Could you check a few things on this model? Use its own coordinates, in mm. A direction names the side the tool comes from. Give positions to 0.01 mm unless a question says otherwise; leave off trailing zeros. Write each loop counter-clockwise with the first axis right and the second up, starting at its lowest first coordinate (ties: lowest second). Pieces come first, ordered by that corner, then holes. Notation, with made-up numbers: M -17,72 L 4,72 A8 ccw 4,80 Z; hole C 78.5,-14.75 d7. An arc over 180 degrees is marked long. Use one line per item in the form item = value.
from build123d import *

# Parameters (mm, degrees)
F0_R       = 53.975
F1_DEPTH   = 590.55
F3_R       = 38.1
F4_DEPTH   = 47.752
F1_FACE_R  = 53.975
F4_FACE_R  = 38.1
F1_FACE1_R = 53.975
F5_FACE_R  = 38.1
F8_SCALE   = 1.6


with BuildPart() as f1:
    # F0 (on Right) → F1 (new body, symmetric)
    with BuildSketch(Plane.YZ):
        Circle(F0_R)
    extrude(amount=F1_DEPTH, both=True)



with BuildPart() as f4:
    # F3 (on offset) → F4 (new body)
    with BuildSketch(Plane.YZ.offset(771.398)):
        Circle(F3_R)
    extrude(amount=-F4_DEPTH)


with BuildPart() as f5_1:
    # F5: instance of F4
    add(f4.part.mirror(Plane.YZ))


with BuildPart() as f1_1:
    add(f1.part)

    add(f4.part)  # F6 merges F4
    # F1_face (on face) → F6 section 0
    with BuildSketch(Plane.YZ.offset(590.55)):
        Circle(F1_FACE_R)
    # F4_face (on face) → F6 section 1
    with BuildSketch(Plane(origin=(723.646, 0, 0), x_dir=(0, 1, 0), z_dir=(-1, 0, 0))):
        Circle(F4_FACE_R)
    loft()


    add(f5_1.part)  # F7 merges F5_1
    # F1_face1 (on face) → F7 section 0
    with BuildSketch(Plane(origin=(-590.55, 0, 0), x_dir=(0, 1, 0), z_dir=(-1, 0, 0))):
        Circle(F1_FACE1_R)
    # F5_face (on face) → F7 section 1
    with BuildSketch(Plane.YZ.offset(-723.646)):
        Circle(F5_FACE_R)
    loft()


with BuildPart() as f1_2:
    # F8: moved
    add(f1_1.part.scale(F8_SCALE))


solid = f1_2.part
1) For faces 1 (the flat face through (-1234.237, -1, 1)), 2 (the cylindrical face through (1196.57, -13.21, -59.51)), 3 (the cylindrical face through (-1196.57, -13.21, -59.51)), which set-ups out of +Z, -Z, +X, -X, +Y, -Y let a thin tool reach every point of the face, with its end or its side?
Checked values:
face_1 = +Z, -Z, -X, +Y, -Y
face_2 = +X
face_3 = -X
2) For pin 1 Ø3 at (x, z) = (370, -43.5) entering from +Y; pin 2 Ø1 at (x, y) = (506, -5) entering from +Z; pin 3 Ø6 at (x, z) = (-39, -8.5) entering from +Y, each with a flat end and sliding along its axis, tell me the tip position at first contact or that it passes through.
Checked values:
pin_1 = 75.46
pin_2 = 86.24
pin_3 = 86.18
3) I want a section at A-A, the plane y = 0. Please give me the cut outline in (x, z).
Checked values:
outline = M -1234.24,-60.96 L -1157.83,-60.96 L -944.88,-86.36 L 944.88,-86.36 L 1157.83,-60.96 L 1234.24,-60.96 L 1234.24,60.96 L 1157.83,60.96 L 944.88,86.36 L -944.88,86.36 L -1157.83,60.96 L -1234.24,60.96 Z
4) I want a section at B-B, the plane x = 846. Please give me the cut outline in (y, z).
Checked values:
outline = C 0,0 d172.72
5) If I drill on L1, parallel to Z at x = 667, y = 8; L2, parallel to Z at x = 1084.5, y = 5; L3, parallel to Y at x = -429, z = 46, over which ranges is the centre line in solid material (lowest first)?
Checked values:
L1 = -85.99 to 85.99
L2 = -69.53 to 69.53
L3 = -73.09 to 73.09
